The model under review builds one solid part; all positions refer to its coordinate system, in mm. A direction names the side the tool comes from. Give positions to 0.01 mm unless a question says otherwise; leave off trailing zeros. Order: outer loops, then holes, each group sorted by start corner. A loop starts at its lowest first (then second) coordinate and runs counter-clockwise, first axis right, second up. Notation, with made-up numbers: (54.5, -32) - (83.5, -32) arc R24 ccw to (83.5, -6) - close; hole circle Ø1 at (-7.75, 35). An arc over 180 degrees is marked (long way). Use CSV: the item, a comma, the result in double quotes. Start each with the question number.
```python
from build123d import *

# Parameters (mm, degrees)
F1_DEPTH = 5
F4_DEPTH = 3.5


with BuildPart() as f1:
    # F0 (on Top) → F1 (new body)
    with BuildSketch(Plane.XY):
        with BuildLine():
            add(Edge.make_bspline(
                [(-25.2, 12), (-24.770263451, 13.7320665567), (-22.5559362307, 17.3933294028), (-19.7388011355, 17.4001357259), (-18, 17.6210526316)],
                knots=[0, 0, 0, 0, 0.5263054949, 1, 1, 1, 1], degree=3))
            ThreePointArc((-25.2, 12), (-26.1941368445, 0), (-25.2, -12))
            add(Edge.make_bspline(
                [(-25.2, -12), (-24.770263451, -13.7320665567), (-22.5559362307, -17.3933294028), (-19.7388011355, -17.4001357259), (-18, -17.6210526316)],
                knots=[0, 0, 0, 0, 0.5263054949, 1, 1, 1, 1], degree=3))
            ThreePointArc((-18, -17.6210526316), (0, -18.4210526316), (18, -17.6210526316))
            add(Edge.make_bspline(
                [(25.2, -12), (24.770263451, -13.7320665567), (22.5559362307, -17.3933294028), (19.7388011355, -17.4001357259), (18, -17.6210526316)],
                knots=[0, 0, 0, 0, 0.5263054949, 1, 1, 1, 1], degree=3))
            ThreePointArc((25.2, -12), (26.1941368445, 0), (25.2, 12))
            add(Edge.make_bspline(
                [(25.2, 12), (24.770263451, 13.7320665567), (22.5559362307, 17.3933294028), (19.7388011355, 17.4001357259), (18, 17.6210526316)],
                knots=[0, 0, 0, 0, 0.5263054949, 1, 1, 1, 1], degree=3))
            ThreePointArc((18, 17.6210526316), (0, 18.4210526316), (-18, 17.6210526316))
        make_face()
        Polygon((-5.5, -7.5), (-5.5, 7.5), (8.5, 0), align=None, mode=Mode.SUBTRACT)
    extrude(amount=F1_DEPTH)


with BuildPart() as f1_1:
    # F2: moved
    add(f1.part)

    # F3 (on face) → F4 (cut)
    with BuildSketch(Plane.XY.offset(5)):
        with BuildLine():
            ThreePointArc((-23.302383765, -1.5), (-23.7787077069, 0), (-23.302383765, 1.5))
            Line((-23.302383765, 1.5), (-26.1787077069, 1.5))
            ThreePointArc((-26.1787077069, 1.5), (-26.1941368445, 0), (-26.1787077069, -1.5))
            Line((-26.1787077069, -1.5), (-23.302383765, -1.5))
        make_face()
        with BuildLine():
            ThreePointArc((-23.302383765, -1.5), (-20.3918016614, -2.478059498), (-18.5787077069, 0))
            ThreePointArc((-18.5787077069, 0), (-20.3918016614, 2.478059498), (-23.302383765, 1.5))
            ThreePointArc((-23.302383765, 1.5), (-23.7787077069, 0), (-23.302383765, -1.5))
        make_face()
    extrude(amount=-F4_DEPTH, mode=Mode.SUBTRACT)


solid = f1_1.part
```
1. Consider section C-C (y = -11). Give the boundary of the cut face in (x, z).
2. Consider section A-A (x = 0.5). Give the boundary of the cut face in (y, z).
3. To check wall thickness, follow L1, parallel to X at y = 4, z = 1.4; L2, parallel to X at y = 7, z = 3.1; L3, parallel to Y at x = 4, z = 1.1. State the ranges of each line that lie inside material, in increasing order. Write a range as [from, to].
4. Mouldability with a two-part tool opening along X and no side actions: class faces 1 (the face through (-5.5, 0, 2)), 2 (the face through (0.25, 18.42, 2.46)), 3 (the face through (6, 4, 0)), 4 (the face through (-22, 0, 1.5)) as pulls with the +X half, pulls with the -X half, needs draft (parallel to the pull), parting line crosses it, or undercut.
5. Tool access review of faces 5 (the face through (6, 4, 5)), 6 (the face through (-25, -1.5, 3)), 7 (the face through (1.402, 3.802, 2.465)): name each direction out of +Z, -Z, +X, -X, +Y, -Y from which nothing blocks a thin tool from reaching the whole face with its end or side.
6. Consider section B-B (x = 12.5). Give the boundary of the cut face in (y, z).
7. Clearance check with flat-ended pins moving along their axes: pin 1 (3 mm diameter, centred on x = -2.5, z = 3, fed in from -Y); pin 2 (2 mm diameter, centred on y = -6.5, z = 3, fed in from -X); pin 3 (2 mm diameter, centred on y = 12, z = 3, fed in from +X). State where each tip first meets the part, or that it passes through.
Answers follow:
1,outline,"(-25.36, 0) - (25.36, 0) - (25.36, 5) - (-25.36, 5) - close"
2,outline,"(-18.42, 0) - (-4.29, 0) - (-4.29, 5) - (-18.42, 5) - close; (4.29, 0) - (18.42, 0) - (18.42, 5) - (4.29, 5) - close"
3,L1,"x = [-26.08, -5.5], [1.03, 26.08]"
3,L2,"x = [-25.86, -5.5], [-4.57, 25.86]"
3,L3,"y = [-18.38, -2.41], [2.41, 18.38]"
4,face 1,"undercut"
4,face 2,"parting line crosses it"
4,face 3,"needs draft"
4,face 4,"undercut"
5,face 5,"+Z, +X, -X, +Y, -Y"
5,face 6,"+Z, -X"
5,face 7,"+Z, -Z"
6,outline,"(-18.04, 0) - (18.04, 0) - (18.04, 5) - (-18.04, 5) - close"
7,pin 1,"stops at y = -18.42"
7,pin 2,"stops at x = -25.99"
7,pin 3,"stops at x = 25.36"
